Geometry: final body of the model. Coordinates: model frame, mm. Face numbers are marked on the shaded views. A direction names the side the tool comes from. Round coordinates to 2 decimals unless told otherwise and drop trailing zeros. Write each loop counter-clockwise with the first axis right and the second up, starting at its lowest first coordinate (ties: lowest second). Pieces come first, ordered by that corner, then holes. Notation, with made-up numbers: (7.25, 73) -> (20.25, 73) arc R10 ccw to (20.25, 79) -> close; hole circle Ø8 at (49, -8.75). An arc over 180 degrees is marked (long way). Use one line per item in the form item = value. Start each with the question number.
1. Pin query (flat end, axial travel): pin 1 Ø1.5 at (y, z) = (-19, -39) entering from +X; pin 2 Ø3 at (x, z) = (-11.5, -39) entering from -Y; pin 3 Ø4 at (y, z) = (30, 0.5) entering from +X. Return the tip coordinate at first contact, or that it passes through.
2. Cut plane C-C, the plane z = -34. Return the cut outline in (x, y).
3. Reachability of the marked faces 1, 2 and 3 from +Z, -Z, +X, -X, +Y, -Y: full face, straight path, thin tool, end or side. Return the list, or none.
4. Cut plane A-A, the plane y = 0. Return the cut outline in (x, z).
5. Cut plane D-D, the plane z = 48.5. Return the cut outline in (x, y).
6. Line query: L1, parallel to Z at x = 13, y = 31.5; L2, parallel to Z at x = -8, y = -29; L3, parallel to Y at x = 38, z = 12. Output: solid intervals per line, ascending.
```python
from build123d import *

# Parameters (mm, degrees)
F0_R     = 51
F1_DEPTH = 42.5
F2_R     = 17.5
F3_R     = 24.5
F4_DEPTH = 17.8
F5_R     = 1
F6_DEPTH = 42.5
F7_R     = 33
F8_DEPTH = 11


# Not quite as in the source:
# - a feature of the source that left no trace in its solid (it failed there, or was rolled back) is left out


with BuildPart() as f1:
    # F0 (on Top) → F1 (new body)
    with BuildSketch(Plane.XY):
        Circle(F0_R)
    extrude(amount=F1_DEPTH)

    # F2
    f2_edges = [f1.edges().sort_by_distance(p)[0] for p in [
        (-51, 0, 42.5),
    ]]
    fillet(f2_edges, radius=F2_R)

    # F3 (on face) → F4 (join)
    with BuildSketch(Plane.XY.offset(42.5)):
        Circle(F3_R)
    extrude(amount=F4_DEPTH)

    # F5
    f5_edges = [f1.edges().sort_by_distance(p)[0] for p in [
        (-24.5, 0, 60.3),
    ]]
    fillet(f5_edges, radius=F5_R)

    # F6 (add): a face of the model
    f6_faces = [f1.faces().sort_by_distance(p)[0] for p in [
        (0, 0, 0),
    ]]
    extrude(f6_faces, amount=F6_DEPTH)

    # F7 (on face) → F8 (join)
    with BuildSketch(Plane(origin=(0, 0, -42.5), x_dir=(1, 0, 0), z_dir=(0, 0, -1))):
        Circle(F7_R)
    extrude(amount=F8_DEPTH)


solid = f1.part
```
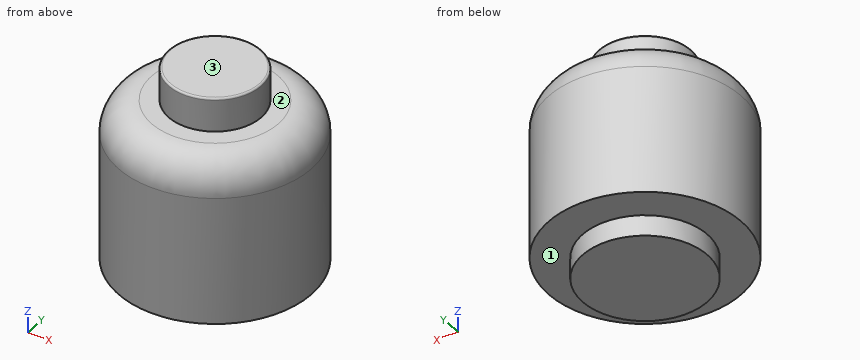
Outcome:
q1.pin_1 = 47.62
q1.pin_2 = -50.01
q1.pin_3 = 42.63
q2.outline = circle Ø102 at (0, 0)
q3.face_1 = -Z
q3.face_2 = +Z
q3.face_3 = +Z, +X, -X, +Y, -Y
q4.outline = (-51, -42.5) -> (-33, -42.5) -> (-33, -53.5) -> (33, -53.5) -> (33, -42.5) -> (51, -42.5) -> (51, 25) arc R17.5 ccw to (33.5, 42.5) -> (24.5, 42.5) -> (24.5, 59.3) arc R1 ccw to (23.5, 60.3) -> (-23.5, 60.3) arc R1 ccw to (-24.5, 59.3) -> (-24.5, 42.5) -> (-33.5, 42.5) arc R17.5 ccw to (-51, 25) -> close
q5.outline = circle Ø49 at (0, 0)
q6.L1 = -42.5 to 42.49
q6.L2 = -53.5 to 42.5
q6.L3 = -34.01 to 34.01
